Can you work these out from the model? Positions are in its coordinate system, mm. A direction names the side the tool comes from. Coordinates: 2 decimals unless noted, no trailing zeros. Order: outer loops, then holes, each group sorted by start corner. A loop starts at its lowest first (then second) coordinate and runs counter-clockwise, first axis right, second up. Notation, with made-up numbers: (59, 26) -> (102, 26) arc R19 cw to (102, 46) -> close; hole circle Ø9 at (53.5, 41.5). An arc over 180 degrees is marked (long way). Return JSON: item names as keys, results as strings. Group by question number.
1) For pin 1 (12 mm diameter, centred on x = 12, z = 238.5, fed in from +Y); pin 2 (4 mm diameter, centred on x = 5.5, z = 261.5, fed in from +Y); pin 3 (10 mm diameter, centred on x = 7, z = 221, fed in from +Y), each with a flat end and sliding along its axis, tell me the tip position at first contact or that it passes through.
2) If we section it at A-A, the plane z = 207: Please give me the cut outline in (x, y) (3 decimals), then the cut area to 3 significant figures.
3) If we section it at C-C, the plane x = 21: Please give me the cut outline in (y, z) (3 decimals), then the cut area to 3 significant figures.
4) For faces 1 (the flat face through (15, 3.175, 155)), 2 (the flat face through (0, 13, 156)), which set-ups out of +Z, -Z, +X, -X, +Y, -Y let a thin tool reach every point of the face, with its end or its side?
5) If we section it at B-B, the plane y = 14: Please give me the cut outline in (x, z) (3 decimals).
6) If I drill on probe 1 along X at (y, z) = (21.75, 79.5) (3 decimals); probe 2 along Z at (x, y) = (2.75, 10.75), over which ranges is the centre line in solid material (lowest first)? Write a range as from..to.
Autodesk Inventor part; units mm, degrees
ref_plane "Start Plane" through (0, 0, 24.5) normal (0, 0, 1) x (1, 0, 0)
ref_plane "End Plane" through (0, 0, 290.1887) normal (0, 0, 1) x (1, 0, 0)
ref_plane "Work Plane4" through (0, 12.7, 290.1887) normal (0.018, 0, 0.9998) x (0.9998, 0, -0.018)
ref_plane "Start Plane" through (0, 0, 24.5) normal (0, 0, 1) x (1, 0, 0)
ref_plane "End Plane" through (0, 0, 290.1887) normal (0, 0, 1) x (1, 0, 0)
sketch "Sketch" plane through (0, 0, 0) normal (0, 0, 1) x (1, 0, 0)
  line L0 (25.4, 0) -> (0, 0)
  line L1 (0, 0) -> (0, 25.4)
  line L2 (0, 25.4) -> (1.651, 25.4)
  line L3 (3.175, 23.876) -> (3.175, 6.477)
  line L4 (6.477, 3.175) -> (23.876, 3.175)
  line L5 (25.4, 1.651) -> (25.4, 0)
  line L6 (0, -11.0414) -> (0, 31.5385) construction
  line L7 (-11.0414, 0) -> (31.5385, 0) construction
  arc A0 (3.175, 6.477) -> (6.477, 3.175) centre (6.477, 6.477) ccw
  arc A1 (3.175, 23.876) -> (1.651, 25.4) centre (1.651, 23.876) ccw
  arc A2 (25.4, 1.651) -> (23.876, 3.175) centre (23.876, 1.651) ccw
  line L8 (0, 40.0545) -> (0, -19.5574) construction
  line L9 (-19.5574, 0) -> (40.0545, 0) construction
  point P0 (3.175, 25.4)
  point P1 (3.175, 3.175)
  point P2 (25.4, 3.175)
  dimension "d0" = 25.4
  dimension "d1" = 25.4
  dimension "d2" = 3.175
  dimension "d3" = 3.175
  dimension "d10" = 0
  dimension "d11" = 0
  dimension "d14" = 3.302
  dimension "d15" = 1.524
extrude "Body" add sketch "Sketch" along normal up to surface (265.6887 mm away) from surface at 24.5
sketch "Sketch3" plane through (0, 0, 0) normal (0, 0, 1) x (1, 0, 0)
  line L0 (0, 0) -> (10, 0)
ref_plane "Work Plane3" through (0, 0, 0) normal (0, -1, 0) x (1, 0, 0)
ref_plane "Work Plane4" through (0, 12.7, 290.1887) normal (0.018, 0, 0.9998) x (0.9998, 0, -0.018)
split "Split1" plane through (0, 12.7, 290.1887) removes the side toward (0.018, 0, 0.9998)
ref_plane "Work Plane9" through (0.9159, 690, 25.3835) normal (-0.0361, 0, -0.9993) x (-0.9993, 0, 0.0361)
split "Split3" plane through (0.9159, 690, 25.3835) removes the side toward (-0.0361, 0, -0.9993)
sketch "Sketch4" plane through (0, 0, 0) normal (0, -1, 0) x (1, 0, 0)
  line L0 (-2, 24.5) -> (12, 24.5)
  line L1 (-2, 290.1887) -> (12, 290.1887)
  dimension "d17" = 265.6887
equation "\"d0\" = G_H"
equation "\"d1\" = G_H"
equation "\"d2\" = G_T"
equation "\"d3\" = G_T"
equation "\"d14\" = G_IR"
equation "\"d15\" = G_ER"
equation "\"d4\" = G_L"
equation "\"G_H\" = 25.4"
equation "\"G_T\" = 3.175"
equation "\"G_ER\" = 1.524"
equation "\"G_IR\" = 3.302"
equation "\"G_L\" = 265.69027"
equation "\"ex\" = 0"
equation "\"G_OFFSET_START\" = -24.50003"
equation "\"G_OFFSET_END\" = 0"
equation "\"d12\" = -G_OFFSET_START"
equation "\"d13\" = G_OFFSET_END + B_L"
equation "\"B_L\" = 290.18872"
properties part number "AISC - L 1 x 1 x 1/8 - 10.46" material "Steel, Mild"
Result sheet:
{
 "1": {"pin 1": "stops at y = 3.21", "pin 2": "stops at y = 5.05", "pin 3": "stops at y = 25.36"},
 "2": {"outline": "(0, 0) -> (25.4, 0) -> (25.4, 1.651) arc R1.524 ccw to (23.876, 3.175) -> (6.477, 3.175) arc R3.302 cw to (3.175, 6.477) -> (3.175, 23.876) arc R1.524 ccw to (1.651, 25.4) -> (0, 25.4) -> close", "area": "153 mm2"},
 "3": {"outline": "(0, 24.658) -> (3.175, 24.658) -> (3.175, 289.811) -> (0, 289.811) -> close", "area": "842 mm2"},
 "4": {"face 1": "+Z, -Z, +X, +Y", "face 2": "+Z, -Z, -X, +Y, -Y"},
 "5": {"outline": "(0, 25.417) -> (3.175, 25.302) -> (3.175, 290.132) -> (0, 290.189) -> close"},
 "6": {"probe 1": "x = 0..3.175", "probe 2": "z = 25.32..290.14"}
}
